```python
from build123d import *

# Parameters (mm, degrees)
SKETCH_1_W          = 44
SKETCH_1_H          = 4.5
SKETCH_1_W_2        = 3
SKETCH_1_H_2        = 7
SKETCH_1_H_3        = 3
SKETCH_5_W          = 39
SKETCH_5_H          = 1
CUT_EXTRUDE_2_DEPTH = 5


with BuildPart() as part:
    # 草圖1 → 旋轉1 (revolve)
    with BuildSketch(Plane.XY):
        with Locations((-22, 2.25)):
            Rectangle(SKETCH_1_W, SKETCH_1_H)
        with Locations((1.5, 3.5)):
            Rectangle(SKETCH_1_W_2, SKETCH_1_H_2)
        with Locations((4.5, 1.5)):
            Rectangle(SKETCH_1_W_2, SKETCH_1_H_3)
    revolve(axis=Axis((0, 0, 0), (-1, 0, 0)))

    # 草圖5 → 除料-伸長2 (cut, symmetric)
    with BuildSketch(Plane.XY):
        with Locations((-24.5, 4)):
            Rectangle(SKETCH_5_W, SKETCH_5_H)
        with Locations((-24.5, -4)):
            Rectangle(SKETCH_5_W, SKETCH_5_H)
    extrude(amount=CUT_EXTRUDE_2_DEPTH, both=True, mode=Mode.SUBTRACT)


solid = part.part
```
Verification items for the finished model (mm, model axes). A direction names the side the tool comes from. Give positions to 0.01 mm unless a question says otherwise; leave off trailing zeros. Loops run counter-clockwise (first coordinate to the right, second up) from the corner with the lowest first, then second, coordinate; pieces in that order, holes last. Notation, with made-up numbers: M 11.5,-20 L 66.5,-20 A34 ccw 66.5,16 Z; hole C 27,73.25 d9. An arc over 180 degrees is marked long. Return JSON: item names as keys, results as strings.
1) Section check D-D, the plane x = -37. Enter the section's corners in (y, z).
Findings:
{"outline": "M -3.5,-2.83 A4.5 ccw 3.5,-2.83 L 3.5,2.83 A4.5 ccw -3.5,2.83 Z"}
2) Section check A-A, the plane z = 0. Enter the section's corners in (x, y), and give its area (3 significant figures).
Findings:
{"outline": "M -44,-3.5 L -5,-3.5 L -5,-4.5 L 0,-4.5 L 0,-7 L 3,-7 L 3,-3 L 6,-3 L 6,3 L 3,3 L 3,7 L 0,7 L 0,4.5 L -5,4.5 L -5,3.5 L -44,3.5 Z", "area": "378 mm2"}
3) Tool access check on faces 1 (the flat face through (-25, 3.5, 0)), 2 (the flat face through (6, 0, 0)), 3 (the flat face through (-5, -4, 0)), 4 (the cylindrical face through (-21.69, -0.59, -4.46)), 5 (the cylindrical face through (5, -3, 0)). Record the directions out of +Z, -Z, +X, -X, +Y, -Y that give a thin tool (end or side, any length) a straight path to the whole face; none if there is none.
Findings:
{"face 1": "+Z, -Z, -X, +Y", "face 2": "+Z, -Z, +X, +Y, -Y", "face 3": "+Z, -Z, -X, -Y", "face 4": "-X", "face 5": "+X"}
4) Material ranges on L1, parallel to Y at x = -12.5, z = 0.5; L2, parallel to X at y = -3.75, z = -4; L3, parallel to X at y = 1, z = 3.5, recorded low to high. Write a range as [from, to].
Findings:
{"L1": "y = [-3.5, 3.5]", "L2": "x = [0, 3]", "L3": "x = [-44, 3]"}
5) Section check B-B, the plane y = 0. Enter the section's corners in (x, z), and give its area (3 significant figures).
Findings:
{"outline": "M -44,-4.5 L 0,-4.5 L 0,-7 L 3,-7 L 3,-3 L 6,-3 L 6,3 L 3,3 L 3,7 L 0,7 L 0,4.5 L -44,4.5 Z", "area": "456 mm2"}
6) Section check C-C, the plane x = 2. Enter the section's corners in (y, z), and give its area (3 significant figures).
Findings:
{"outline": "C 0,0 d14", "area": "154 mm2"}
7) Gauge pin test, flat ends, axial feed: P1, Ø3, axis at x = -18, z = 0.5, coming from the -Y side; P2, Ø3, axis at x = -38.5, y = 2, coming from the -Z side; P3, Ø3, axis at x = -23.5, z = 0.5, coming from the +Y side. Record the tip position at first contact, or that the pin passes through.
Findings:
{"P1": "stops at y = -3.5", "P2": "stops at z = -4.47", "P3": "stops at y = 3.5"}
